Here's how the part is built. I have some questions about the finished solid (model axes, mm). Give positions to 0.01 mm unless a question says otherwise; leave off trailing zeros. Write each loop counter-clockwise with the first axis right and the second up, starting at its lowest first coordinate (ties: lowest second). Pieces come first, ordered by that corner, then holes. Notation, with made-up numbers: (87.25, -29) -> (142.25, -29) arc R8 cw to (142.25, -16) -> close; hole circle Ø5 at (-33, 76). An arc over 180 degrees is marked (long way). Use one line per item in the form item = value.
```python
from build123d import *

# Parameters (mm, degrees)
SKETCH1_R           = 1.25
BOSS_EXTRUDE1_DEPTH = 6
SKETCH3_R           = 4.75
BOSS_EXTRUDE3_DEPTH = 0.77
FILLET1_R           = 0.7
SKETCH4_W           = 0.63
SKETCH4_H           = 9.781785326
CUT_EXTRUDE1_DEPTH  = 0.5


with BuildPart() as part:
    # Sketch1 → Boss-Extrude1 (new body)
    with BuildSketch(Plane(origin=(0, 0, 0), x_dir=(1, 0, 0), z_dir=(0, 1, 0))):
        with Locations(Location((0, 0, 0), (0, 0, 270))):
            Circle(SKETCH1_R)
    extrude(amount=BOSS_EXTRUDE1_DEPTH)

    # Sketch3 → Boss-Extrude3 (add)
    with BuildSketch(Plane.XZ):
        with Locations(Location((0, 0, 0), (0, 0, 270))):
            Circle(SKETCH3_R)
    extrude(amount=BOSS_EXTRUDE3_DEPTH)

    # Fillet1
    fillet1_edges = [part.edges().sort_by_distance(p)[0] for p in [
        (0, -0.77, 4.75),
    ]]
    fillet(fillet1_edges, radius=FILLET1_R)

    # Sketch4 → Cut-Extrude1 (cut)
    with BuildSketch(Plane.XZ.offset(0.77)):
        Rectangle(SKETCH4_W, SKETCH4_H)
    extrude(amount=-CUT_EXTRUDE1_DEPTH, mode=Mode.SUBTRACT)


solid = part.part
```
Q1. Will this pin go through, and if not, where does the flat tip stop? pin 1 Ø1.5 at (x, z) = (2.5, -2) entering from +Y.
Result set:
pin_1 = 0
Q2. I want a section at A-A, the plane z = 0. Write out the boundary of the cut face in (x, y) (3 decimals).
Result set:
outline = (-4.75, -0.07) arc R0.7 ccw to (-4.05, -0.77) -> (-0.315, -0.77) -> (-0.315, -0.27) -> (0.315, -0.27) -> (0.315, -0.77) -> (4.05, -0.77) arc R0.7 ccw to (4.75, -0.07) -> (4.75, 0) -> (1.25, 0) -> (1.25, 6) -> (-1.25, 6) -> (-1.25, 0) -> (-4.75, 0) -> close
Q3. I want a section at B-B, the plane x = 0. Write out the boundary of the cut face in (y, z), and give its area (3 significant figures).
Result set:
outline = (-0.27, -4.72) arc R0.7 ccw to (-0.07, -4.75) -> (0, -4.75) -> (0, -1.25) -> (6, -1.25) -> (6, 1.25) -> (0, 1.25) -> (0, 4.75) -> (-0.07, 4.75) arc R0.7 ccw to (-0.27, 4.72) -> close
area = 17.6 mm2
Q4. I want a section at C-C, the plane y = 0.5. Write out the boundary of the cut face in (x, z), and give its area (3 significant figures).
Result set:
outline = circle Ø2.5 at (0, 0)
area = 4.91 mm2
Q5. If I drill on line 1 along Y through (x, z) = (2.75, -2.5); line 2 along Y through (x, z) = (0, -2); line 3 along X through (y, z) = (0.25, -0.75), over which ranges is the centre line in solid material (lowest first)? Write a range as from..to.
Result set:
line_1 = -0.77..0
line_2 = -0.27..0
line_3 = -1..1
Q6. If we mould it in two halves opening along Y, with no side actions, what happens to faces 1 (the face through (-1, 0, -1)), 2 (the face through (-1.22, 2.96, -0.27)), 3 (the face through (-2, -0.77, 0))? For each: +Y half, -Y half, draft (parallel to the pull), parting line (faces both ways), or undercut.
Result set:
face_1 = +Y half
face_2 = draft
face_3 = -Y half
